The model under review builds one solid part; all positions refer to its coordinate system, in mm. Face numbers are marked on the shaded views. A direction names the side the tool comes from. Coordinates: 2 decimals unless noted, no trailing zeros. Write each loop counter-clockwise with the first axis right and the second up, starting at its lowest first coordinate (ties: lowest second). Pieces come first, ordered by that corner, then holes. Notation, with made-up numbers: (-31, 46.5) - (15, 46.5) arc R27 cw to (15, 75.5) - close; hole circle Ø2 at (-4, 44.25). An arc over 180 degrees is marked (long way). Put each result on its own line as item: value. Start each with the question number.
Item 1: Consider section A-A on z = 5. Give the boundary of the cut face in (x, y).
Item 2: Consider section D-D on y = 1. Give the boundary of the cut face in (x, z).
Item 3: Mouldability with a two-part tool opening along Z and no side actions: class the marked faces 3, 4, 5 and 6 as pulls with the +Z half, pulls with the -Z half, needs draft (parallel to the pull), parting line crosses it, or undercut.
Item 4: For pin 1 (3.5 mm diameter, centred on y = 11.5, z = 5, fed in from -X), flat-tipped, find the tip position at first contact; note if it passes through.
Item 5: Consider section B-B on y = -2.5. Give the boundary of the cut face in (x, z).
Item 6: To check wall thickness, follow L1, parallel to Y at x = -0.9, z = 5; L2, parallel to Z at x = -4.75, y = -15.7; L3, parallel to Z at x = -1.75, y = 3. State the ranges of each line that lie inside material, in increasing order. Write a range as [from, to].
Item 7: Consider section C-C on x = -4.75. Give the boundary of the cut face in (y, z), then the cut area to 3 significant figures.
Item 8: Machinability: for the marked faces 1 and 2, which of the approach directions +Z, -Z, +X, -X, +Y, -Y give a long, thin tool a straight path to every point of the face, cutting with its end or side? Answer none if there is none.
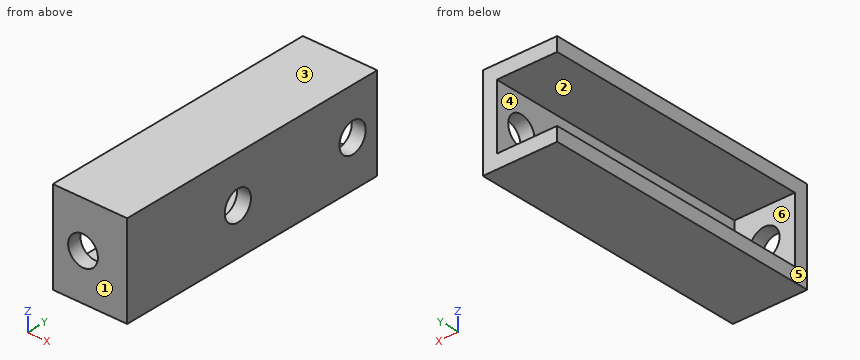
Autodesk Inventor part; units mm, degrees
ref_plane "YZ Plane" through (0, 0, 0) normal (1, 0, 0) x (0, 1, 0)
ref_plane "XZ Plane" through (0, 0, 0) normal (0, 1, 0) x (-1, 0, 0)
ref_plane "XY Plane" through (0, 0, 0) normal (0, 0, 1) x (1, 0, 0)
sketch "Náčrt1" plane through (0, 0, 0) normal (0, 1, 0) x (-1, 0, 0)
  line L0 (0, -2) -> (0, 12)
  line L1 (-1.6, 0) -> (9.6, 0)
  line L2 (8, 10) -> (0, 10)
  line L3 (0, 10) -> (0, 0)
  line L4 (0, 0) -> (8, 0)
  line L5 (8, 0) -> (8, 10)
  line L6 (8, 8.5) -> (1.5, 8.5)
  line L7 (1.5, 8.5) -> (1.5, 1.5)
  line L8 (1.5, 1.5) -> (8, 1.5)
  line L9 (8, 1.5) -> (8, 8.5)
  point P0 (0, 0)
  point P1 (0, 10)
  dimension "d0" = 8
  dimension "d1" = 10
  dimension "d2" = 6.5
  dimension "d3" = 7
  dimension "d4" = 1.5
extrude "Vysunutí1" add sketch "Náčrt1" along normal mid plane 29 contours L0 L2 L5 L6 L7 L8 L1
sketch "Náčrt2" plane through (0, -14.5, 0) normal (0, -1, 0) x (1, 0, 0)
  line L0 (-8, 8.5) -> (-1.5, 8.5)
  line L1 (-1.5, 8.5) -> (-1.5, 1.5)
  line L2 (-1.5, 1.5) -> (-8, 1.5)
  line L3 (-8, 1.5) -> (-8, 0)
  line L4 (-8, 0) -> (0, 0)
  line L5 (0, 0) -> (0, 10)
  line L6 (0, 10) -> (-8, 10)
  line L7 (-8, 10) -> (-8, 8.5)
  line L8 (-8, 10) -> (0, 10)
  line L9 (0, 10) -> (0, 0)
  line L10 (0, 0) -> (-8, 0)
  line L11 (-8, 0) -> (-8, 10)
extrude "Vysunutí2" add sketch "Náčrt2" along normal blind 1.5
sketch "Náčrt3" plane through (0, -14.5, 0) normal (0, 1, 0) x (1, 0, 0)
  line L0 (-8, -8.5) -> (-1.5, -8.5)
  line L1 (-1.5, -8.5) -> (-1.5, -1.5)
  line L2 (-1.5, -1.5) -> (-8, -1.5)
  line L3 (-8, -8.5) -> (-8, -1.5)
  point P0 (0, 0)
  point P1 (-4.75, -5)
  dimension "d9" = 3.25
  dimension "d10" = 3.5
hole "Díra1" at (-4.75, -14.5, 5) direction (0, -1, 0) diameter 3.2 end through all
sketch "Náčrt4" plane through (-1.5, 14.5, 1.5) normal (-1, 0, 0) x (0, 0, 1)
  line L0 (0, 0) -> (7, 0)
  line L1 (7, 0) -> (7, -29)
  line L2 (0, 0) -> (7, 0)
  line L3 (0, -29) -> (0, 0)
  line L4 (7, -29) -> (0, -29)
  point P0 (-1.5, -14.5)
  point P1 (3.5, -3)
  point P2 (3.5, -17)
  point P3 (3.5, 0)
  dimension "d18" = 3
  dimension "d19" = 14
  dimension "d20" = 3.5
  dimension "d21" = 3.5
hole "Díra2" at (-1.5, 11.5, 5) at (-1.5, -2.5, 5) direction (1, 0, 0) diameter 3.2 end through all
properties part number "lift_tab_bracket" material "Hliník 6061"
Report:
1. outline: (-8, -16) - (-6.35, -16) - (-6.35, -14.5) - (-8, -14.5) - close; (-3.15, -16) - (0, -16) - (0, -4.1) - (-1.5, -4.1) - (-1.5, -14.5) - (-3.15, -14.5) - close; (-1.5, -0.9) - (0, -0.9) - (0, 9.9) - (-1.5, 9.9) - close; (-1.5, 13.1) - (0, 13.1) - (0, 14.5) - (-1.5, 14.5) - close
2. outline: (-8, 0) - (0, 0) - (0, 10) - (-8, 10) - (-8, 8.5) - (-1.5, 8.5) - (-1.5, 1.5) - (-8, 1.5) - close
3. face 3: pulls with the +Z half
3. face 4: undercut
3. face 5: needs draft
3. face 6: undercut
4. pin 1: x = -1.5
5. outline: (-8, 0) - (0, 0) - (0, 3.4) - (-1.5, 3.4) - (-1.5, 1.5) - (-8, 1.5) - close; (-8, 8.5) - (-1.5, 8.5) - (-1.5, 6.6) - (0, 6.6) - (0, 10) - (-8, 10) - close
6. L1: [-16, -4.1], [-0.9, 9.9], [13.1, 14.5]
6. L2: [0, 3.4], [6.6, 10]
6. L3: [0, 1.5], [8.5, 10]
7. outline: (-16, 0) - (14.5, 0) - (14.5, 1.5) - (-14.5, 1.5) - (-14.5, 3.4) - (-16, 3.4) - close; (-16, 6.6) - (-14.5, 6.6) - (-14.5, 8.5) - (14.5, 8.5) - (14.5, 10) - (-16, 10) - close
7. area: 97.2 mm²
8. face 1: +Z, -Z, +X, -X, -Y
8. face 2: -X, +Y
